Read the model definition and answer for the solid it produces. Units are mm, in the model's axes. Round coordinates to 2 decimals unless told otherwise and drop trailing zeros. Write each loop counter-clockwise with the first axis right and the second up, starting at its lowest first coordinate (ties: lowest second). Pieces come first, ordered by that corner, then holes.
from build123d import *

# Parameters (mm, degrees)
SKETCH1_R           = 18
SKETCH1_R_2         = 2.12769231
SKETCH1_R_3         = 6.9156293
BOSS_EXTRUDE1_DEPTH = 210


with BuildPart() as part:
    # Sketch1 → Boss-Extrude1 (new body)
    with BuildSketch(Plane(origin=(0, 0, 0), x_dir=(1, 0, 0), z_dir=(0, 1, 0))):
        Circle(SKETCH1_R)
        with Locations((0, 13)):
            Circle(SKETCH1_R_2, mode=Mode.SUBTRACT)
        Circle(SKETCH1_R_3, mode=Mode.SUBTRACT)
        with Locations((11.258330249, 6.5)):
            Circle(SKETCH1_R_2, mode=Mode.SUBTRACT)
        with Locations((11.258330249, -6.5)):
            Circle(SKETCH1_R_2, mode=Mode.SUBTRACT)
        with Locations((0, -13)):
            Circle(SKETCH1_R_2, mode=Mode.SUBTRACT)
        with Locations((-11.258330249, -6.5)):
            Circle(SKETCH1_R_2, mode=Mode.SUBTRACT)
        with Locations((-11.258330249, 6.5)):
            Circle(SKETCH1_R_2, mode=Mode.SUBTRACT)
    extrude(amount=BOSS_EXTRUDE1_DEPTH)


solid = part.part
Q1. Determine the mould class of faces 1 (the flat face through (0, 0, 8)), 2 (the cylindrical face through (-2.343, 103.53, -17.847)), 3 (the cylindrical face through (-13.384, 103.53, 6.406)) for opening direction X: pulls with the +X half, pulls with the -X half, needs draft (parallel to the pull), parting line crosses it, or undercut.
Verdict:
face 1: needs draft
face 2: parting line crosses it
face 3: undercut
Q2. Flat-ended cylindrical pins translate along their axes: pin 1 Ø1.5 at (x, y) = (-2.5, 100) entering from -Z; pin 2 Ø2.5 at (x, z) = (0, 13) entering from -Y; pin 3 Ø1 at (y, z) = (165, 1) entering from +X; pin 4 Ø1 at (y, z) = (110.5, -3) entering from -X. Find the tip coordinate at first contact, or state that the pin passes through.
Verdict:
pin 1: stops at z = -17.91
pin 2: passes through
pin 3: stops at x = 17.99
pin 4: stops at x = -17.83
Q3. Straight lines are drawn through the part: probe 1 along Z at (x, y) = (12, 88.5); probe 2 along Z at (x, y) = (0, 136.5); probe 3 along Z at (x, y) = (11, 25). For each, find the intervals that lie inside material, in ascending order.
Verdict:
probe 1: z = -13.42 to -8.49, -4.51 to 4.51, 8.49 to 13.42
probe 2: z = -18 to -15.13, -10.87 to -6.92, 6.92 to 10.87, 15.13 to 18
probe 3: z = -14.25 to -8.61, -4.39 to 4.39, 8.61 to 14.25
Q4. Section C-C (z = -13) is taken. Determine the outline of the cut face in (x, y).
Verdict:
outline: (-12.45, 0) - (-2.13, 0) - (-2.13, 210) - (-12.45, 210) - close; (2.13, 0) - (12.45, 0) - (12.45, 210) - (2.13, 210) - close
Q5. Section A-A (y = 46.5) is taken. Determine the outline of the cut face in (x, z), then the cut area to 3 significant figures.
Verdict:
outline: circle Ø36 at (0, 0); hole circle Ø4.26 at (-11.26, -6.5); hole circle Ø4.26 at (-11.26, 6.5); hole circle Ø13.83 at (0, 0); hole circle Ø4.26 at (0, -13); hole circle Ø4.26 at (0, 13); hole circle Ø4.26 at (11.26, -6.5); hole circle Ø4.26 at (11.26, 6.5)
area: 782 mm2
Q6. Section B-B (x = 0) is taken. Determine the outline of the cut face in (y, z).
Verdict:
outline: (0, -18) - (210, -18) - (210, -15.13) - (0, -15.13) - close; (0, -10.87) - (210, -10.87) - (210, -6.92) - (0, -6.92) - close; (0, 6.92) - (210, 6.92) - (210, 10.87) - (0, 10.87) - close; (0, 15.13) - (210, 15.13) - (210, 18) - (0, 18) - close
